Work out the finished part from the listing and answer in its coordinate system (mm). Coordinates: 2 decimals unless noted, no trailing zeros. Loops run counter-clockwise (first coordinate to the right, second up) from the corner with the lowest first, then second, coordinate; pieces in that order, holes last. Notation, with made-up numbers: M 1.25,6.5 L 60.25,6.5 A30 cw 60.25,39.5 Z; hole C 23.5,-30.5 d10. An arc over 180 degrees is marked long. Write each question's results on one line, items separated by ' | '.
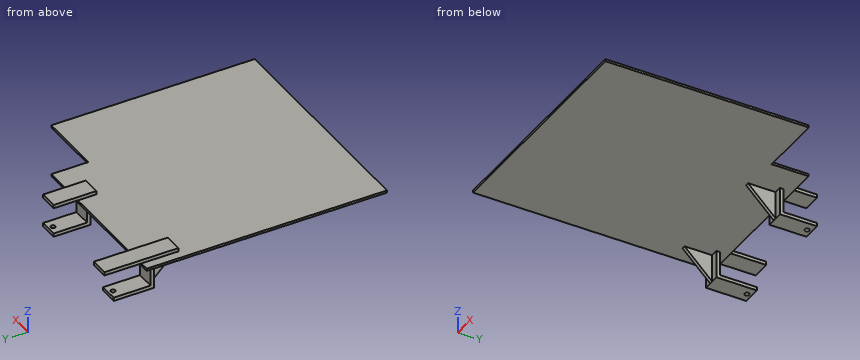
```python
from build123d import *

# Parameters (mm, degrees)
F1_DEPTH  = 6.35
F2_W      = 50.8
F2_H      = 101.6
F3_DEPTH  = 9.525
F4_W      = 50.8
F4_H      = 9.525
F5_DEPTH  = 76.2
F6_W      = 50.8
F6_H      = 9.525
F7_DEPTH  = 92.075
F8_R      = 6.35
F9_DEPTH  = 25.4
F10_W     = 50.8
F10_H     = 66.675
F10_H_2   = 50.8
F11_DEPTH = 9.525
F12_W     = 9.525
F12_H     = 76.2
F13_DEPTH = 76.2
F15_DEPTH = 25.4
F16_W     = 50.8
F16_H     = 9.525
F17_DEPTH = 76.2
F18_W     = 50.8
F18_H     = 9.525
F19_DEPTH = 101.6
F20_R     = 6.35
F21_DEPTH = 25.4
F22_W     = 9.525
F22_H     = 76.2
F23_DEPTH = 76.2
F25_DEPTH = 25.4


with BuildPart() as f1:
    # F0 (on Top) → F1 (new body)
    with BuildSketch(Plane.XY):
        Polygon((-317.5, -330.2), (317.5, -330.2), (317.5, 228.6), (139.7, 228.6), (139.7, 330.2), (-317.5, 330.2), align=None)
    extrude(amount=F1_DEPTH)

    # F2 (on face) → F3 (join)
    with BuildSketch(Plane.XY.offset(6.35)):
        with Locations((-266.7, 279.4)):
            Rectangle(F2_W, F2_H)
        with Locations((-266.7, 381)):
            Rectangle(F2_W, F2_H)
    extrude(amount=F3_DEPTH)

    # F4 (on face) → F5 (join)
    with BuildSketch(Plane(origin=(0, 0, 0), x_dir=(1, 0, 0), z_dir=(0, 0, -1))):
        with Locations((38.1, -300.0375)):
            Rectangle(F4_W, F4_H)
    extrude(amount=F5_DEPTH)

    # F6 (on face) → F7 (join)
    with BuildSketch(Plane(origin=(0, 304.8, 0), x_dir=(-1, 0, 0), z_dir=(0, 1, 0))):
        with Locations((-38.1, -71.4375)):
            Rectangle(F6_W, F6_H)
    extrude(amount=F7_DEPTH)

    # F8 (on face) → F9 (cut)
    with BuildSketch(Plane(origin=(0, 0, -76.2), x_dir=(1, 0, 0), z_dir=(0, 0, -1))):
        with Locations((38.1, -384.175)):
            Circle(F8_R)
    extrude(amount=-F9_DEPTH, mode=Mode.SUBTRACT)

    # F10 (on face) → F11 (join)
    with BuildSketch(Plane.XY.offset(6.35)):
        with Locations((38.1, 363.5375)):
            Rectangle(F10_W, F10_H)
        with Locations((38.1, 304.8)):
            Rectangle(F10_W, F10_H_2)
    extrude(amount=F11_DEPTH)

    # F12 (on face) → F13 (join)
    with BuildSketch(Plane.XZ.offset(-295.275)):
        with Locations((38.1, -38.1)):
            Rectangle(F12_W, F12_H)
    extrude(amount=F13_DEPTH)

    # F14 (on face) → F15 (cut)
    with BuildSketch(Plane.YZ.offset(42.8625)):
        Polygon((219.075, -76.2), (295.275, -76.2), (219.075, 0), align=None)
    extrude(amount=-F15_DEPTH, mode=Mode.SUBTRACT)

    # F16 (on face) → F17 (join)
    with BuildSketch(Plane(origin=(0, 0, 0), x_dir=(1, 0, 0), z_dir=(0, 0, -1))):
        with Locations((-266.7, -300.0375)):
            Rectangle(F16_W, F16_H)
    extrude(amount=F17_DEPTH)

    # F18 (on face) → F19 (join)
    with BuildSketch(Plane(origin=(0, 304.8, 0), x_dir=(-1, 0, 0), z_dir=(0, 1, 0))):
        with Locations((266.7, -71.4375)):
            Rectangle(F18_W, F18_H)
    extrude(amount=F19_DEPTH)

    # F20 (on face) → F21 (cut)
    with BuildSketch(Plane(origin=(0, 0, -76.2), x_dir=(1, 0, 0), z_dir=(0, 0, -1))):
        with Locations((-266.7, -393.7)):
            Circle(F20_R)
    extrude(amount=-F21_DEPTH, mode=Mode.SUBTRACT)

    # F22 (on face) → F23 (join)
    with BuildSketch(Plane.XZ.offset(-295.275)):
        with Locations((-266.7, -38.1)):
            Rectangle(F22_W, F22_H)
    extrude(amount=F23_DEPTH)

    # F24 (on face) → F25 (cut)
    with BuildSketch(Plane(origin=(-271.4625, 0, 0), x_dir=(0, -1, 0), z_dir=(-1, 0, 0))):
        Polygon((-219.075, 0), (-295.275, -76.2), (-219.075, -76.2), align=None)
    extrude(amount=-F25_DEPTH, mode=Mode.SUBTRACT)


solid = f1.part
```
1) Find section D-D, the plane x = 271. Give the vertices of the cut face in (y, z), and give its area (3 significant figures).
Check result:
outline: M -330.2,0 L 228.6,0 L 228.6,6.35 L -330.2,6.35 Z | area: 3,550 mm^2
2) Find section B-B, the plane x = 53.5. Give the vertices of the cut face in (y, z) (3 decimals).
Check result:
outline: M -330.2,0 L 295.275,0 L 295.275,-76.2 L 396.875,-76.2 L 396.875,-66.675 L 304.8,-66.675 L 304.8,0 L 330.2,0 L 330.2,6.35 L 396.875,6.35 L 396.875,15.875 L 279.4,15.875 L 279.4,6.35 L -330.2,6.35 Z
3) Find section C-C, the plane y = -247.5. Give the vertices of the cut face in (x, z).
Check result:
outline: M -317.5,0 L 317.5,0 L 317.5,6.35 L -317.5,6.35 Z
4) Find section A-A, the plane z = -41. Give the vertices of the cut face in (x, y) (1 decimal), and give its area (3 significant figures).
Check result:
outline: M -292.1,295.3 L -271.5,295.3 L -271.5,260.1 L -261.9,260.1 L -261.9,295.3 L -241.3,295.3 L -241.3,304.8 L -292.1,304.8 Z; M 12.7,295.3 L 33.3,295.3 L 33.3,260.1 L 42.9,260.1 L 42.9,295.3 L 63.5,295.3 L 63.5,304.8 L 12.7,304.8 Z | area: 1,640 mm^2
5) Given pin 1 Ø5 at (y, z) = (372, 12.5) entering from +X; pin 2 Ø3 at (x, z) = (166, 6.5) entering from +Y; pin 3 Ø3 at (x, z) = (-167.5, 2.5) entering from +Y; pin 4 Ø23 at (y, z) = (245.5, -51) entering from +X, each flat-ended and moving along its own axis, determine where each tip first touches the part or whether it passes through.
Check result:
pin 1: x = 63.5 | pin 2: y = 228.6 | pin 3: y = 330.2 | pin 4: through
6) Straight lines are drawn through the part: probe 1 along X at (y, z) = (393.7, -70.5); probe 2 along Z at (x, y) = (251.5, -230); probe 3 along Y at (x, z) = (38.1, -69.25) (3 decimals). For each, find the intervals that lie inside material, in ascending order. Write a range as [from, to].
Check result:
probe 1: [-292.1, -273.05], [-260.35, -241.3], [12.7, 63.5] | probe 2: [0, 6.35] | probe 3: [288.325, 377.825], [390.525, 396.875]
